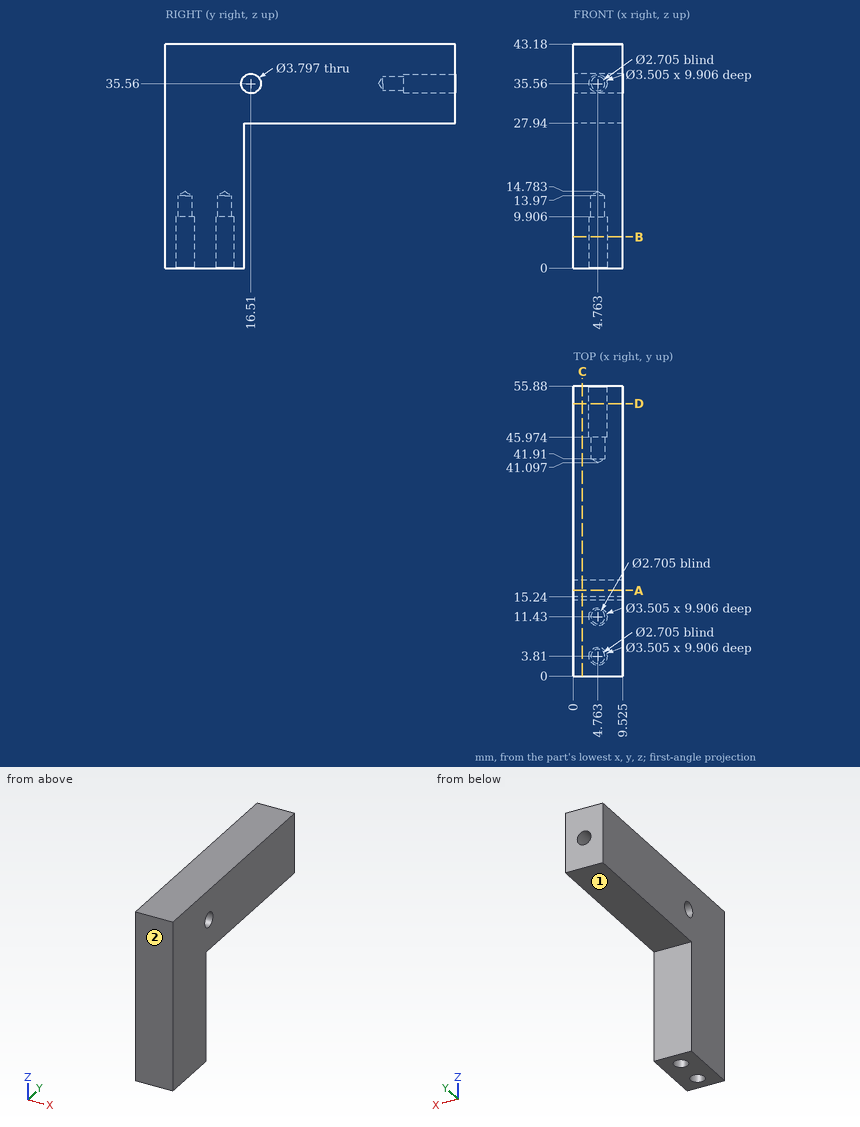
Geometry: see drawing. Coordinates: mm, zero at the bounding-box minimum. A direction names the side the tool comes from. Coordinates: 2 decimals unless noted, no trailing zeros. Loops run counter-clockwise (first coordinate to the right, second up) from the corner with the lowest first, then second, coordinate; pieces in that order, holes last.
(1) Section C-C on x = 1.75. Return the cut outline in (y, z).
(2) Set-up query: the marked faces 1 and 2. Return all of +Z, -Z, +X, -X, +Y, -Y with unobstructed straight access to the full face (end or side cutting, diameter ignored); none if empty.
(3) Section B-B on z = 6. Return the cut outline in (x, y) (1 decimal), then the cut area to 3 significant figures.
(4) Material intervals for probe 1 along Z at (x, y) = (4.75, 16.51); probe 2 along Y at (x, z) = (8, 14.5); probe 3 along Z at (x, y) = (8.75, 30.5), sorted ascending.
(5) Section D-D on y = 52.5. Return the cut outline in (x, z) (1 decimal).
(6) First-contact query: pin 1 Ø1.1 at (x, z) = (4, 36) entering from +Y; pin 2 Ø1.1 at (x, y) = (4.5, 3.5) entering from -Z; pin 3 Ø1.1 at (x, y) = (4, 11) entering from -Z. Flat tips, straight axial feed; report the tip coordinate or a pass-through.
(7) Section A-A on y = 16.51. Return the cut outline in (x, z) (1 decimal), then the cut area to 3 significant figures.
Data:
1. outline: (0, 0) - (15.24, 0) - (15.24, 27.94) - (55.88, 27.94) - (55.88, 43.18) - (0, 43.18) - close; hole circle Ø3.8 at (16.51, 35.56)
2. face 1: -Z, +X, -X, +Y
2. face 2: +Z, -Z, +X, -X, -Y
3. outline: (0, 0) - (9.5, 0) - (9.5, 15.2) - (0, 15.2) - close; hole circle Ø3.5 at (4.8, 3.8); hole circle Ø3.5 at (4.8, 11.4)
3. area: 126 mm2
4. probe 1: z = 27.94 to 33.66, 37.46 to 43.18
4. probe 2: y = 0 to 15.24
4. probe 3: z = 27.94 to 43.18
5. outline: (0, 27.9) - (9.5, 27.9) - (9.5, 43.2) - (0, 43.2) - close; hole circle Ø3.5 at (4.8, 35.6)
6. pin 1: stops at y = 45.97
6. pin 2: stops at z = 14.21
6. pin 3: stops at z = 9.91
7. outline: (0, 27.9) - (9.5, 27.9) - (9.5, 33.7) - (0, 33.7) - close; (0, 37.5) - (9.5, 37.5) - (9.5, 43.2) - (0, 43.2) - close
7. area: 109 mm2
